```python
from build123d import *

# Parameters (mm, degrees)
SKETCH2_R          = 29
SKETCH2_R_2        = 25
SKETCH3_R          = 27
SKETCH3_R_2        = 25
CUT_EXTRUDE1_DEPTH = 5
SKETCH4_R          = 27
SKETCH4_R_2        = 25
CUT_EXTRUDE2_DEPTH = 5


with BuildPart() as part:
    # Sweep1: sweep along a path in Sketch1
    with BuildLine(Plane.XY) as sweep1_path:
        Line((-20, 30), (0, 30))
        ThreePointArc((0, 30), (21.213203436, 21.213203436), (30, 0))
        Line((30, 0), (30, -20))
    # Sketch2 → Sweep1 (sweep)
    with BuildSketch(Plane(origin=(0, -20, 0), x_dir=(1, 0, 0), z_dir=(0, 1, 0))):
        with Locations((30, 0)):
            Circle(SKETCH2_R)
        with Locations((30, 0)):
            Circle(SKETCH2_R_2, mode=Mode.SUBTRACT)
    sweep(path=sweep1_path.line)

    # Sketch3 → Cut-Extrude1 (cut)
    with BuildSketch(Plane.ZY.offset(20)):
        with Locations((0, 30)):
            Circle(SKETCH3_R)
        with Locations((0, 30)):
            Circle(SKETCH3_R_2, mode=Mode.SUBTRACT)
    extrude(amount=-CUT_EXTRUDE1_DEPTH, mode=Mode.SUBTRACT)

    # Sketch4 → Cut-Extrude2 (cut)
    with BuildSketch(Plane.XZ.offset(20)):
        with Locations((30, 0)):
            Circle(SKETCH4_R)
        with Locations((30, 0)):
            Circle(SKETCH4_R_2, mode=Mode.SUBTRACT)
    extrude(amount=-CUT_EXTRUDE2_DEPTH, mode=Mode.SUBTRACT)


solid = part.part
```
The listing builds one solid part. Answer for the finished solid, in the listing's coordinates (mm). A direction names the side the tool comes from. Give positions to 0.01 mm unless a question says otherwise; leave off trailing zeros. Loops run counter-clockwise (first coordinate to the right, second up) from the corner with the lowest first, then second, coordinate; pieces in that order, holes last. Notation, with made-up numbers: (-14.5, 58.25) - (0.5, 58.25) arc R23 cw to (0.5, 69.25) - close; hole circle Ø2 at (65.25, 66.25). An arc over 180 degrees is marked (long way). Return JSON: item names as keys, results as strings. Group by question number.
1. Which of the six approach directions +Z, -Z, +X, -X, +Y, -Y give full straight-line access (tool end or side, diameter ignored) to faces 1 (the flat face through (-20, 38, -26)), 2 (the cylindrical face through (-17.54, 56.77, -3.51)), 3 (the flat face through (38, -15, -24))?
2. Straight lines are drawn through the part: line 1 (X direction, y = -9.75, z = 0); line 2 (Z direction, x = 30, y = -16.4); line 3 (Z direction, x = -7.5, y = 30). For each, find the intervals that lie inside material, in ascending order. Write a range as [from, to].
3. Find section A-A (z = 0). Write down the section's boundary in (x, y), then the cut area to 3 significant figures.
4. Given pin 1 Ø5 at (y, z) = (7.5, 13.5) entering from +X; pin 2 Ø8 at (x, z) = (20.5, -20) entering from -Y; pin 3 Ø4 at (x, z) = (-1.5, 22.5) entering from -Y, each flat-ended and moving along its own axis, determine where each tip first touches the part or whether it passes through.
5. Determine the mould class of faces 4 (the cylindrical face through (-9.86, 6.99, -17.65)), 5 (the flat face through (4, -20, 8)), 6 (the cylindrical face through (11.574, -7.605, 16.896)) for opening direction Z: pulls with the +Z half, pulls with the -Z half, needs draft (parallel to the pull), parting line crosses it, or undercut.
6. Find section B-B (z = 20). Write down the section's boundary in (x, y), then the cut area to 3 significant figures.
Verdict:
{
 "1": {"face 1": "+Z, -Z, -X, +Y, -Y", "face 2": "-X", "face 3": "-Y"},
 "2": {"line 1": "x = [1, 5], [55, 59]", "line 2": "z = [-29, -27], [27, 29]", "line 3": "z = [-29, -25], [25, 29]"},
 "3": {"outline": "(-20, 1) - (0, 1) arc R1 cw to (1, 0) - (1, -20) - (3, -20) - (3, -15) - (5, -15) - (5, 0) arc R5 ccw to (0, 5) - (-15, 5) - (-15, 3) - (-20, 3) - close; (-20, 57) - (-15, 57) - (-15, 55) - (0, 55) arc R55 cw to (55, 0) - (55, -15) - (57, -15) - (57, -20) - (59, -20) - (59, 0) arc R59 ccw to (0, 59) - (-20, 59) - close", "area": "657 mm^2"},
 "4": {"pin 1": "stops at x = 56.38", "pin 2": "stops at y = -15", "pin 3": "stops at y = 9.49"},
 "5": {"face 4": "parting line crosses it", "face 5": "needs draft", "face 6": "undercut"},
 "6": {"outline": "(-20, 9) - (0, 9) arc R9 cw to (9, 0) - (9, -20) - (11.86, -20) - (11.86, -15) - (15, -15) - (15, 0) arc R15 ccw to (0, 15) - (-15, 15) - (-15, 11.86) - (-20, 11.86) - close; (-20, 48.14) - (-15, 48.14) - (-15, 45) - (0, 45) arc R45 cw to (45, 0) - (45, -15) - (48.14, -15) - (48.14, -20) - (51, -20) - (51, 0) arc R51 ccw to (0, 51) - (-20, 51) - close", "area": "983 mm^2"}
}
